Build history of the part. All positions in model axes, mm. Face numbers are marked on the shaded views. A direction names the side the tool comes from. Coordinates: 2 decimals unless noted, no trailing zeros. Order: outer loops, then holes, each group sorted by start corner. A loop starts at its lowest first (then second) coordinate and runs counter-clockwise, first axis right, second up. Notation, with made-up numbers: (9.5, 3) - (57.5, 3) arc R25 ccw to (57.5, 22) - close; hole circle Ø10 at (53, 42). An arc over 180 degrees is marked (long way). One line per item, written item: value.
Autodesk Inventor part; units mm, degrees
ref_plane "YZ Plane" through (0, 0, 0) normal (1, 0, 0) x (0, 1, 0)
ref_plane "XZ Plane" through (0, 0, 0) normal (0, 1, 0) x (-1, 0, 0)
ref_plane "XY Plane" through (0, 0, 0) normal (0, 0, 1) x (1, 0, 0)
sketch "Sketch1" plane through (0, 0, 0) normal (0, 1, 0) x (-1, 0, 0)
  line L0 (0, 0) -> (40, 0)
  line L1 (40, 0) -> (40, -40)
  line L2 (40, -40) -> (0, -40)
  line L3 (0, -40) -> (0, 0)
  line L4 (2, -2) -> (38, -2)
  line L5 (38, -2) -> (38, -38)
  line L6 (38, -38) -> (2, -38)
  line L7 (2, -38) -> (2, -2)
  dimension "d0" = 40
  dimension "d1" = 40
  dimension "d2" = 2
  dimension "d3" = 2
  dimension "d4" = 2
  dimension "d5" = 2
extrude "Extrusion1" add sketch "Sketch1" along normal blind 4 contours L4 L5 L6 L7
extrude "Extrusion2" add sketch "Sketch1" along normal blind 60
sketch "Sketch2" plane through (0, 4, 0) normal (0, 1, 0) x (1, 0, 0)
  line L0 (-26.995, 38) -> (-13.005, 38)
  line L1 (-11.1, 36.095) -> (-11.1, 18.905)
  line L2 (-13.005, 17) -> (-26.995, 17)
  line L3 (-28.9, 18.905) -> (-28.9, 36.095)
  arc A0 (-26.995, 38) -> (-28.9, 36.095) centre (-26.995, 36.095) ccw
  arc A1 (-11.1, 36.095) -> (-13.005, 38) centre (-13.005, 36.095) ccw
  arc A2 (-28.9, 18.905) -> (-26.995, 17) centre (-26.995, 18.905) ccw
  arc A3 (-13.005, 17) -> (-11.1, 18.905) centre (-13.005, 18.905) ccw
  line L4 (-38, 38) -> (-2, 38)
  line L5 (-38, 2) -> (-38, 38)
  line L6 (-30.4, 36.095) -> (-30.4, 18.905)
  arc A4 (-30.4, 18.905) -> (-26.995, 15.5) centre (-26.995, 18.905) ccw
  line L7 (-26.995, 15.5) -> (-13.005, 15.5)
  arc A5 (-13.005, 15.5) -> (-9.6, 18.905) centre (-13.005, 18.905) ccw
  line L8 (-9.6, 18.905) -> (-9.6, 36.095)
  arc A6 (-9.6, 36.095) -> (-10.1828, 38) centre (-13.005, 36.095) ccw
  arc A7 (-29.8172, 38) -> (-30.4, 36.095) centre (-26.995, 36.095) ccw
  line L9 (-29.8172, 38) -> (-10.1828, 38)
  line L10 (-40, 40) -> (-40, 0)
  point P0 (0, 0)
  point P1 (-11.1, 17)
  point P2 (-11.1, 38)
  point P3 (-28.9, 17)
  point P4 (-20, 38)
  point P5 (-13.005, 38)
  point P6 (-20, 17)
  dimension "d11" = 17.8
  dimension "d12" = 21
  dimension "d13" = 1.905
  dimension "d14" = 0
  dimension "d16" = 1.5
  dimension "d25" = 20
extrude "Extrusion3" add sketch "Sketch2" along normal blind 1.2 contours A0 L3 A2 L2 A3 L1 A1 L4 A6 L8 A5 L7 A4 L6 A7
sketch "Sketch3" plane through (-38, 60, -38) normal (0, 0, 1) x (1, 0, 0)
  point P0 (38, -60)
sketch "Sketch4" plane through (0, 0, -40) normal (0, 0, -1) x (-1, 0, 0)
  line L0 (16.35, 6.9) -> (23.65, 6.9) construction
  line L1 (16.35, 4.7) -> (23.65, 4.7)
  line L2 (23.65, 9.1) -> (16.35, 9.1)
  arc A0 (16.35, 9.1) -> (16.35, 4.7) centre (16.35, 6.9) ccw
  arc A1 (23.65, 4.7) -> (23.65, 9.1) centre (23.65, 6.9) ccw
  line L3 (0, 0) -> (40, 0)
  line L4 (0, 0) -> (0, 60)
  point P0 (20, 6.9)
  dimension "d19" = 7.3
  dimension "d20" = 4.4
  dimension "d21" = 4.7
  dimension "d22" = 20
extrude "Extrusion4" cut sketch "Sketch4" against normal blind 2
properties part number "sensor_block" material "Brass, Soft Yellow, Welded"
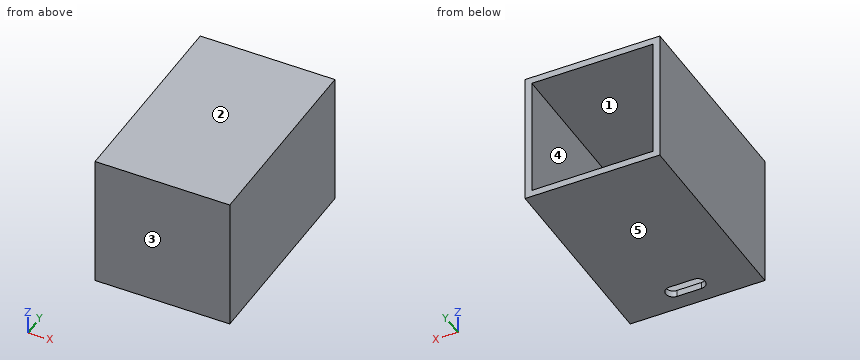
1. Probe line 1 along X through (y, z) = (39.5, -6); line 2 along Y through (x, z) = (-23, -24). List the from-to ranges inside material, lowest first.
Values found:
line 1: x = -40 to -38, -2 to 0
line 2: y = 0 to 4
2. Band-saw the part on C-C, the plane x = -3. Give the cut face in (y, z), and give its area (3 significant figures).
Values found:
outline: (0, -40) - (60, -40) - (60, -38) - (4, -38) - (4, -2) - (60, -2) - (60, 0) - (0, 0) - close
area: 384 mm2
3. Flat gauge pins, fed straight in: P1, Ø9, axis at x = -16, z = -31, coming from the +Y side; P2, Ø0.6, axis at x = -19.5, z = -39, coming from the -Y side; P3, Ø10, axis at x = -25, z = -23, coming from the +Y side. Where does each tip first touch, or does it go through?
Values found:
P1: stops at y = 4
P2: stops at y = 0
P3: stops at y = 5.2
4. 3-axis set-ups, long thin cutter, end or side, ignore diameter. For the marked faces 1 and 2: which of +Z, -Z, +X, -X, +Y, -Y reach the whole face in a straight line?
Values found:
face 1: +Y
face 2: +Z, +X, -X, +Y, -Y
5. Two-plate mould, pull along Z, no slides. Class the marked faces 3, 4 and 5: pulls with the +Z half, pulls with the -Z half, needs draft (parallel to the pull), parting line crosses it, or undercut.
Values found:
face 3: needs draft
face 4: undercut
face 5: pulls with the -Z half
6. Band-saw the part on A-A, the plane y = 28.5. Give the cut face in (x, z), and give its area (3 significant figures).
Values found:
outline: (-40, -40) - (0, -40) - (0, 0) - (-40, 0) - close; hole (-38, -38) - (-2, -38) - (-2, -2) - (-38, -2) - close
area: 304 mm2
7. Band-saw the part on B-B, the plane z = -22.5. Give the cut face in (x, y).
Values found:
outline: (-40, 0) - (0, 0) - (0, 60) - (-2, 60) - (-2, 4) - (-9.6, 4) - (-9.6, 5.2) - (-11.1, 5.2) - (-11.1, 4) - (-28.9, 4) - (-28.9, 5.2) - (-30.4, 5.2) - (-30.4, 4) - (-38, 4) - (-38, 60) - (-40, 60) - close
8. Band-saw the part on D-D, the plane y = 6.9. Give the cut face in (x, z).
Values found:
outline: (-40, -40) - (-25.85, -40) - (-25.85, -38) - (-38, -38) - (-38, -2) - (-2, -2) - (-2, -38) - (-14.15, -38) - (-14.15, -40) - (0, -40) - (0, 0) - (-40, 0) - close
